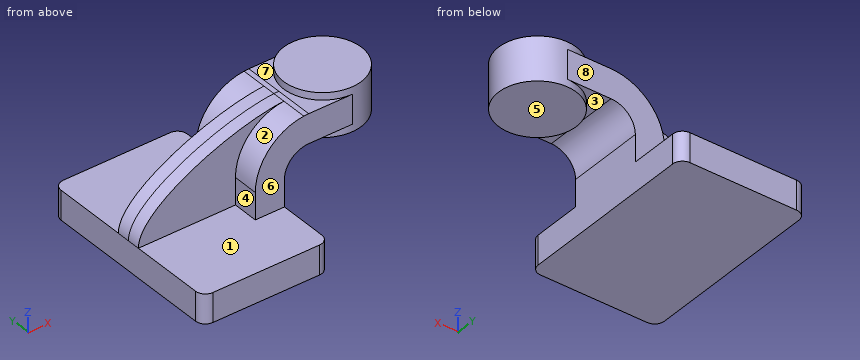
```python
from build123d import *

# Parameters (mm, degrees)
F1_DEPTH = 63.5
F2_DEPTH = 25.4
F3_DEPTH = 8.509
F4_DEPTH = 25.4
F6_R     = 6.35


with BuildPart() as f1:
    # F0 (on Front) → F1 (new body, symmetric)
    with BuildSketch(Plane.XZ):
        Polygon((22.225, 9.525), (-41.275, 9.525), (-41.275, -9.525), (41.275, -9.525), (41.275, 9.525), align=None)
    extrude(amount=F1_DEPTH, both=True)

    # F0 (on Front) → F2 (join, symmetric)
    with BuildSketch(Plane.XZ):
        with BuildLine():
            Line((22.225, 27.0002), (22.225, 9.525))
            Line((22.225, 9.525), (41.275, 9.525))
            Line((41.275, 9.525), (41.275, 27.0002))
            ThreePointArc((41.275, 27.0002), (45.92468, 38.22552), (57.15, 42.8752))
            Line((57.15, 42.8752), (60.325, 42.8752))
            Line((60.325, 42.8752), (60.325, 61.9252))
            Line((60.325, 61.9252), (57.15, 61.9252))
            add(Edge.make_bspline(
                [(53.953536, 61.778616), (55.045402, 61.851231), (56.111784, 61.900361), (57.15, 61.9252)],
                knots=[108.105428, 108.105428, 108.105428, 108.105428, 111.504536, 111.504536, 111.504536, 111.504536], degree=3))
            ThreePointArc((53.953536, 61.778616), (31.348913, 50.53867), (22.225, 27.0002))
        make_face()
    extrude(amount=F2_DEPTH, both=True)

    # F0 (on Front) → F3 (join, symmetric)
    with BuildSketch(Plane.XZ):
        with BuildLine():
            add(Edge.make_bspline(
                [(-41.275, 9.525), (-41.275, 33.404525), (19.227765, 59.46916), (53.953536, 61.778616)],
                knots=[0, 0, 0, 0, 108.105428, 108.105428, 108.105428, 108.105428], degree=3))
            Line((-41.275, 9.525), (22.225, 9.525))
            Line((22.225, 9.525), (22.225, 27.0002))
            ThreePointArc((22.225, 27.0002), (31.348913, 50.53867), (53.953536, 61.778616))
        make_face()
    extrude(amount=F3_DEPTH, both=True)

    # F0 (on Front) → F4 (join, symmetric)
    with BuildSketch(Plane.XZ):
        Polygon((76.154022, 61.9252), (60.325, 61.9252), (60.325, 42.8752), (76.154022, 42.8752), (85.725, 42.8752), (85.725, 61.9252), align=None)
    extrude(amount=F4_DEPTH, both=True)

    # F0 (on Front) → F5 (revolve)
    with BuildSketch(Plane.XZ):
        Polygon((111.125, 66.675), (85.725, 66.675), (85.725, 61.9252), (85.725, 42.8752), (85.725, 38.1), (111.125, 38.1), align=None)
    revolve(axis=Axis((85.725, 0, 52.3875), (0, 0, -1)))

    # F6
    f6_edges = [f1.edges().sort_by_distance(p)[0] for p in [
        (-41.275, 63.5, 0),
        (41.275, 63.5, 0),
        (-41.275, -63.5, 0),
        (41.275, -63.5, 0),
    ]]
    fillet(f6_edges, radius=F6_R)


solid = f1.part
```
Work out the finished part from the listing and answer in its coordinate system (mm). Face numbers are marked on the shaded views. A direction names the side the tool comes from. Coordinates: 2 decimals unless noted, no trailing zeros. Order: outer loops, then holes, each group sorted by start corner. A loop starts at its lowest first (then second) coordinate and runs counter-clockwise, first axis right, second up. Notation, with made-up numbers: M 47,2 L 71,2 A14 cw 71,19 Z; hole C 55,-23 d2. An arc over 180 degrees is marked long. Use CSV: the item, a comma, the result in double quotes.
1) Consider line 1 (Y direction, x = 31.5, z = 47); line 2 (Y direction, x = -26, z = 17.5); line 3 (Z direction, x = -1, y = -56) (3 decimals). Determine where each line is inside the solid, lowest interval first. Write a range as [from, to].
Worked out:
line 1,"y = [-25.4, 25.4]"
line 2,"y = [-8.51, 8.51]"
line 3,"z = [-9.525, 9.525]"
2) Section B-B on x = 75.5 is taken. Write down the section's boundary in (y, z) (3 decimals), plus the area to 3 significant figures.
Worked out:
outline,"M -25.4,42.875 L -23.251,42.875 L -23.251,38.1 L 23.251,38.1 L 23.251,42.875 L 25.4,42.875 L 25.4,61.925 L 23.251,61.925 L 23.251,66.675 L -23.251,66.675 L -23.251,61.925 L -25.4,61.925 Z"
area,"1,410 mm^2"
3) Section C-C on y = -54.5 is taken. Write down the section's boundary in (x, z) (3 decimals), plus the area to 3 significant figures.
Worked out:
outline,"M -41.275,-9.525 L 41.275,-9.525 L 41.275,9.525 L -41.275,9.525 Z"
area,"1,570 mm^2"
4) Flat-ended cylindrical pins translate along their axes: pin 1 Ø8 at (x, y) = (-19.5, -35.5) entering from +Z (3 decimals); pin 2 Ø5 at (x, z) = (93.5, 48) entering from +Y; pin 3 Ø5 at (y, z) = (-16, 36.5) entering from +X. Find the tip coordinate at first contact, or state that the pin passes through.
Worked out:
pin 1,"stops at z = 9.525"
pin 2,"stops at y = 24.85"
pin 3,"stops at x = 106.87"
5) Determine the mould class of the marked faces 1, 2 and 3 for opening direction X: released by +X, released by -X, zero draft, split by the parting line, or undercut.
Worked out:
face 1,"zero draft"
face 2,"released by -X"
face 3,"undercut"
6) For the marked faces 4, 5, 6, 7 and 8, determine the directions among +Z, -Z, +X, -X, +Y, -Y from which every point of the face is accessible in a straight line to the end or side of a thin tool.
Worked out:
face 4,"+Z, -X, -Y"
face 5,"-Z, +X, +Y, -Y"
face 6,"+Z, +X, -X, -Y"
face 7,"+Z, -X"
face 8,"+Z, +X, -X, +Y"
7) Section A-A on z = 1.5 is taken. Write down the section's boundary in (x, y) (3 decimals), plus the area to 3 significant figures.
Worked out:
outline,"M -41.275,-57.15 A6.35 ccw -34.925,-63.5 L 34.925,-63.5 A6.35 ccw 41.275,-57.15 L 41.275,57.15 A6.35 ccw 34.925,63.5 L -34.925,63.5 A6.35 ccw -41.275,57.15 Z"
area,"10,400 mm^2"
